```python
from build123d import *

# Parameters (mm, degrees)
SKETCH1_W           = 5
SKETCH1_H           = 5
BOSS_EXTRUDE1_DEPTH = 2.5
EXTRUDE_THIN1_DEPTH = 0.5
EXTRUDE_THIN2_DEPTH = 0.45
LPATTERN1_COUNT     = 2
LPATTERN1_PITCH     = 2.3
SKETCH4_R           = 1.5
BOSS_EXTRUDE2_DEPTH = 0.05
SKETCH5_R           = 0.197706898
CUT_EXTRUDE2_DEPTH  = 0.5


with BuildPart() as part:
    # Sketch1 → Boss-Extrude1 (new body)
    with BuildSketch(Plane.XY):
        with Locations((2.5, 2.5)):
            Rectangle(SKETCH1_W, SKETCH1_H)
    extrude(amount=BOSS_EXTRUDE1_DEPTH)

    # Sketch2 → Extrude-Thin1 (add, symmetric)
    with BuildSketch(Plane(origin=(2.5, 0, 0), x_dir=(0, 0, -1), z_dir=(1, 0, 0))):
        with BuildLine():
            Line((-1.25, 5), (-0.05, 5))
            ThreePointArc((-0.05, 5), (0.126776695, 5.073223305), (0.2, 5.25))
            Line((0.2, 5.25), (0.2, 5.7))
            Line((0.2, 5.7), (0, 5.7))
            Line((0, 5.7), (0, 5.25))
            ThreePointArc((0, 5.25), (-0.014644661, 5.214644661), (-0.05, 5.2))
            Line((-0.05, 5.2), (-1.25, 5.2))
            Line((-1.25, 5.2), (-1.25, 5))
        make_face()
    extrude(amount=EXTRUDE_THIN1_DEPTH, both=True)

    # Sketch3 → Extrude-Thin2 (add, symmetric)
    with BuildSketch(Plane(origin=(1.35, 0, 0), x_dir=(0, 0, -1), z_dir=(1, 0, 0))):
        with BuildLine():
            Line((-1.25, 0), (-0.05, 0))
            ThreePointArc((-0.05, 0), (0.126776695, -0.073223305), (0.2, -0.25))
            Line((0.2, -0.25), (0.2, -0.7))
            Line((0.2, -0.7), (0, -0.7))
            Line((0, -0.7), (0, -0.25))
            ThreePointArc((0, -0.25), (-0.014644661, -0.214644661), (-0.05, -0.2))
            Line((-0.05, -0.2), (-1.25, -0.2))
            Line((-1.25, -0.2), (-1.25, 0))
        make_face()
    extrude_thin2 = extrude(amount=EXTRUDE_THIN2_DEPTH, both=True)

    # LPattern1: Extrude-Thin2 ×2
    with Locations(*[(i * LPATTERN1_PITCH, 0, 0) for i in range(1, LPATTERN1_COUNT)]):
        add(extrude_thin2)

    # Sketch4 → Boss-Extrude2 (add)
    with BuildSketch(Plane.XY.offset(2.5)):
        with Locations((2.5, 2.5)):
            Circle(SKETCH4_R)
    extrude(amount=BOSS_EXTRUDE2_DEPTH)

    # Sketch5 → Cut-Extrude2 (cut)
    with BuildSketch(Plane.XY.offset(2.55)):
        with Locations((2.5, 3.518700577)):
            Circle(SKETCH5_R)
        Polygon((2.018700577, 3.518700577), (2.5, 3.037401154), (2.981299423, 3.518700577), (3.518700577, 2.981299423), (3.037401154, 2.5), (3.518700577, 2.018700577), (2.981299423, 1.481299423), (2.5, 1.962598846), (2.018700577, 1.481299423), (1.481299423, 2.018700577), (1.962598846, 2.5), (1.481299423, 2.981299423), align=None)
    extrude(amount=-CUT_EXTRUDE2_DEPTH, mode=Mode.SUBTRACT)


solid = part.part
```
Model file for the job. Use its own axes, mm. A direction names the side the tool comes from. Coordinates: 2 decimals unless noted, no trailing zeros. Loops run counter-clockwise (first coordinate to the right, second up) from the corner with the lowest first, then second, coordinate; pieces in that order, holes last. Notation, with made-up numbers: M 32,31.25 L 48,31.25 A24 cw 48,61.25 Z; hole C -37.75,4 d5. An arc over 180 degrees is marked long. Use CSV: the item, a comma, the result in double quotes. Start each with the question number.
1. Tool access for faces 1 (the flat face through (3.7, -0.2, 0.6)), 2 (the flat face through (1, 4, 2.5)), 3 (the flat face through (2.5, 5.2, 0.6)): list every direction of +Z, -Z, +X, -X, +Y, -Y with a clear straight run to the whole face (end or side of a thin tool).
2. Band-saw the part on B-B, the plane x = 3.7. List the corners of the cut face in (y, z), then the cut area to 3 significant figures.
3. Flat gauge pins, fed straight in: pin 1 (1.5 mm diameter, centred on x = 1.5, y = 1.5, fed in from -Z); pin 2 (3 mm diameter, centred on x = 1.5, y = 0, fed in from -Z); pin 3 (0.7 mm diameter, centred on x = 1.5, z = 0.5, fed in from -Y). Where does each tip first touch, or does it go through?
4. Two-plate mould, pull along X, no slides. Class faces 4 (the flat face through (2, 0, 1)), 5 (the flat face through (2, 3, 0)), 6 (the flat face through (3, 3, 2.05)), 7 (the flat face through (5, 2, 1)): pulls with the +X half, pulls with the -X half, needs draft (parallel to the pull), parting line crosses it, or undercut.
5. Band-saw the part on C-C, the plane y = 0.25. List the corners of the cut face in (x, z).
6. Band-saw the part on A-A, the plane z = 0.15. List the corners of the cut face in (x, y).
7. Probe probe 1 along Y at (x, z) = (3.25, 2.3); probe 2 along Z at (x, y) = (3.8, 0.75); probe 3 along Y at (x, z) = (1.3, 1.6). List the from-to ranges inside material, lowest first. Write a range as [from, to].
Entries:
1,face 1,"+Z, +X, -X, -Y"
1,face 2,"+Z"
1,face 3,"+Z, +X, -X, +Y"
2,outline,"M -0.7,-0.2 L -0.25,-0.2 A0.25 ccw 0,0.05 L 0,0 L 5,0 L 5,2.5 L 3.4,2.5 L 3.4,2.55 L 1.6,2.55 L 1.6,2.5 L 0,2.5 L 0,1.25 L -0.2,1.25 L -0.2,0.05 A0.05 cw -0.25,0 L -0.7,0 Z"
2,area,"13.0 mm2"
3,pin 1,"stops at z = 0"
3,pin 2,"stops at z = -0.2"
3,pin 3,"stops at y = -0.2"
4,face 4,"undercut"
4,face 5,"needs draft"
4,face 6,"undercut"
4,face 7,"pulls with the +X half"
5,outline,"M 0,0 L 5,0 L 5,2.5 L 0,2.5 Z"
6,outline,"M 0,0 L 0.9,0 L 0.9,-0.2 L 1.8,-0.2 L 1.8,0 L 3.2,0 L 3.2,-0.2 L 4.1,-0.2 L 4.1,0 L 5,0 L 5,5 L 3,5 L 3,5.2 L 2,5.2 L 2,5 L 0,5 Z"
7,probe 1,"y = [0, 1.75], [2.29, 2.71], [3.25, 5]"
7,probe 2,"z = [0, 2.5]"
7,probe 3,"y = [0, 5]"
